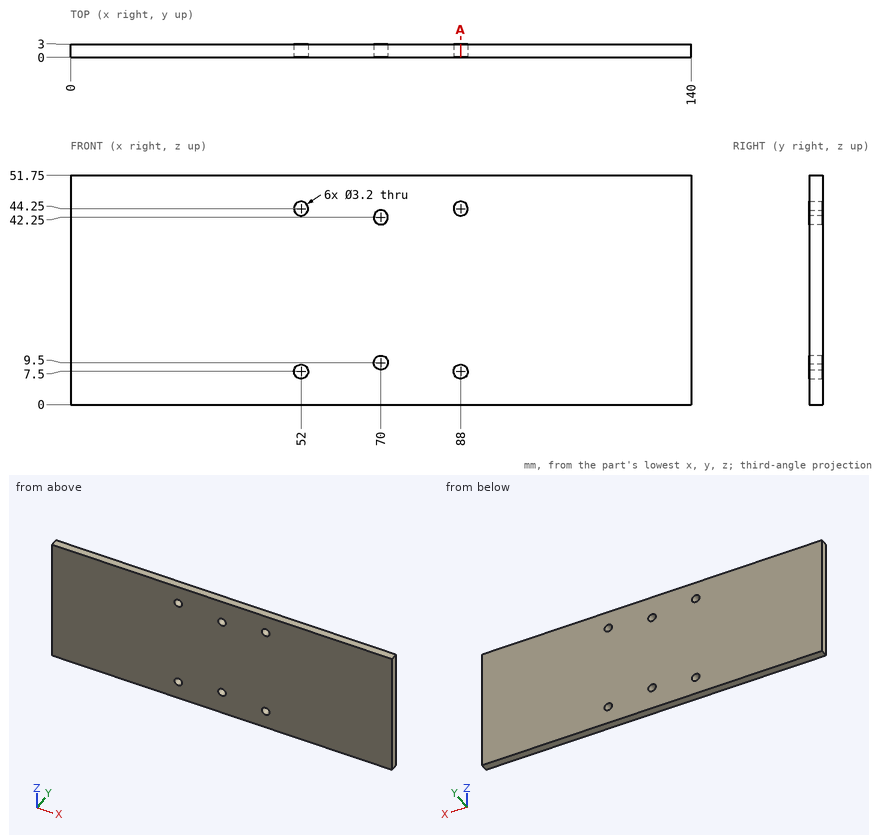
The figure shows three views and two pictorial views of one solid part (mm, origin at its lowest corner). Answer the questions. Give positions to 0.01 mm unless a question says otherwise; leave off trailing zeros. Loops run counter-clockwise (first coordinate to the right, second up) from the corner with the lowest first, then second, coordinate; pieces in that order, holes last. Notation, with made-up numbers: (-38.75, 38) - (5.25, 38) arc R22 cw to (5.25, 51) - close; hole circle Ø8 at (72, -21.5). An arc over 180 degrees is marked (long way). Answer in a Markdown table with one row per item.
(1) Consider L1, parallel to Z at x = 70, y = 1; L2, parallel to X at y = 2, z = 7.5; L3, parallel to X at y = 1.7, z = 9.5. Determine where each line is inside the solid, lowest interval first. Write a range as [from, to].
Results list:
| item | result |
|---|---|
| L1 | z = [0, 7.9], [11.1, 40.65], [43.85, 51.75] |
| L2 | x = [0, 50.4], [53.6, 86.4], [89.6, 140] |
| L3 | x = [0, 68.4], [71.6, 140] |
(2) Section A-A (x = 88) is taken. Give the vertices of the cut face in (y, z).
Results list:
| item | result |
|---|---|
| outline | (0, 0) - (3, 0) - (3, 5.9) - (0, 5.9) - close; (0, 9.1) - (3, 9.1) - (3, 42.65) - (0, 42.65) - close; (0, 45.85) - (3, 45.85) - (3, 51.75) - (0, 51.75) - close |
(3) A flat-ended cylindrical pin translates along its axis: pin 1 Ø1.9 at (x, z) = (70, 42.25) entering from -Y. Find the tip coordinate at first contact, or state that the pin passes through.
Results list:
| item | result |
|---|---|
| pin 1 | passes through |
